Autodesk Inventor part; units mm, degrees
ref_plane "YZ Plane" through (0, 0, 0) normal (1, 0, 0) x (0, 1, 0)
ref_plane "XZ Plane" through (0, 0, 0) normal (0, 1, 0) x (-1, 0, 0)
ref_plane "XY Plane" through (0, 0, 0) normal (0, 0, 1) x (1, 0, 0)
sketch "Sketch1" plane through (0, 0, 0) normal (0, 1, 0) x (-1, 0, 0)
  line L0 (54.6051, -28.5788) -> (-2.5526, -61.5788)
  line L1 (-52.0526, -33) -> (-52.0526, 33)
  line L2 (-2.5526, 61.5788) -> (54.6051, 28.5788)
  circle A0 centre (38.1051, 0) radius 33 construction
  circle A1 centre (-19.0526, 33) radius 33 construction
  circle A2 centre (-19.0526, -33) radius 33 construction
  arc A3 (54.6051, -28.5788) -> (54.6051, 28.5788) centre (38.1051, 0) ccw
  arc A4 (-52.0526, -33) -> (-2.5526, -61.5788) centre (-19.0526, -33) ccw
  arc A5 (-2.5526, 61.5788) -> (-52.0526, 33) centre (-19.0526, 33) ccw
  circle A6 centre (0, 0) radius 3.175
  line L3 (-52.0526, -4.875) -> (-48.6526, -4.875)
  line L4 (-48.6526, -4.875) -> (-40.9371, -1.3266)
  line L5 (-40.9371, 1.3266) -> (-48.6526, 4.875)
  line L6 (-48.6526, 4.875) -> (-52.0526, 4.875)
  arc A7 (-40.9371, -1.3266) -> (-40.9371, 1.3266) centre (-38.0526, 0) ccw
  line L7 (-40.9371, -1.3266) -> (-38.0526, 0) construction
  line L8 (-38.0526, 0) -> (-40.9371, 1.3266) construction
  arc A8 (21.6175, -34.7893) -> (19.3197, -36.1159) centre (19.0263, -32.9545) ccw
  arc A9 (19.3197, 36.1159) -> (21.6175, 34.7893) centre (19.0263, 32.9545) ccw
  circle A10 centre (19.0263, 32.9545) radius 3.175
  circle A11 centre (19.0263, -32.9545) radius 3.175
  point P0 (-52.0526, 0)
  point P1 (-52.0526, 0)
  point P2 (21.6175, -34.7893)
  point P3 (21.6175, 34.7893)
  dimension "d1" = 66
  dimension "d14" = 6.35
  dimension "d15" = 9.75
  dimension "d16" = 3.4
  dimension "d18" = 10.6
  dimension "d20" = 6.35
  dimension "d23" = 360
extrude "Extrusion1" add sketch "Sketch1" along normal blind 9.525 contours L0 A4 L1 L3 L4 A7 L5 L6 A5 L2 A3
sketch "Sketch2" plane through (0, 9.525, 0) normal (0, 1, 0) x (1, 0, 0)
  circle A0 centre (19.0526, -33) radius 28.575
  circle A1 centre (-38.1051, 0) radius 28.575
  circle A2 centre (19.0526, 33) radius 28.575
  circle A3 centre (19.0526, 33) radius 33
  circle A4 centre (-38.1051, 0) radius 33
  circle A5 centre (19.0526, -33) radius 33
  line L0 (-54.6051, -28.5788) -> (2.5526, -61.5788)
  line L1 (2.5526, 61.5788) -> (-54.6051, 28.5788)
  line L2 (52.0526, -33) -> (52.0526, 33)
  point P0 (0, 0)
  point P1 (-99.3426, -2.7496)
  point P2 (47.2901, -87.408)
  point P3 (47.2901, 87.408)
  point P4 (-99.3426, 2.7496)
  point P5 (52.0526, -84.6584)
  point P6 (52.0526, 84.6584)
  dimension "d5" = 57.15
extrude "Extrusion2" cut sketch "Sketch2" against normal blind 5 contours A0 | A1 | A2
fillet "Fillet2" radius 6.35 4 edges at (52.0526, 4.7625, -4.875) (52.0526, 4.7625, 4.875) (40.9371, 4.7625, -1.3266) (40.9371, 4.7625, 1.3266)
properties part number "BOTTOM_PLATE_WEIGHTS_TREBUCHET" material "Wood (Birch)"
For this review, take the finished solid that the model builds, in its own axes (mm). A direction names the side the tool comes from. Coordinates: 2 decimals unless noted, no trailing zeros. Write each loop counter-clockwise with the first axis right and the second up, starting at its lowest first coordinate (ties: lowest second). Pieces come first, ordered by that corner, then holes. Notation, with made-up numbers: (-22, 23) - (-18, 23) arc R28 ccw to (-18, 52) - close; hole circle Ø9 at (33.5, 88). An arc over 180 degrees is marked (long way). Put each result on its own line as item: value.
1. Add section B-B, the plane x = 0. Give the boundary of the cut face in (y, z) (3 decimals), then the cut area to 3 significant figures.
Values found:
outline: (0, -60.105) - (9.525, -60.105) - (9.525, -54.296) - (4.525, -54.296) - (4.525, -11.704) - (9.525, -11.704) - (9.525, -3.175) - (0, -3.175) - close; (0, 3.175) - (9.525, 3.175) - (9.525, 11.704) - (4.525, 11.704) - (4.525, 54.296) - (9.525, 54.296) - (9.525, 60.105) - (0, 60.105) - close
area: 659 mm²
2. Mouldability with a two-part tool opening along X and no side actions: class faces 4 (the cylindrical face through (-66.652, 7.06, -1.256)), 5 (the flat face through (-5, 9.525, 0)), 6 (the flat face through (19, 4.525, 33)), 7 (the flat face through (46.607, 4.696, -3.934)) as released by +X, released by -X, zero draft, split by the parting line, or undercut.
Values found:
face 4: undercut
face 5: zero draft
face 6: undercut
face 7: released by +X
3. Wall thickness on probe 1 along X at (y, z) = (8, 33); probe 2 along Z at (x, y) = (16.5, 8); probe 3 along Z at (x, y) = (10.5, 4.75): over which ranges is each line inside the solid? List them lowest first.
Values found:
probe 1: -46.95 to -22.2, -15.85 to -9.52, 47.63 to 52.05
probe 2: -65.9 to -61.46, -4.54 to 4.54, 61.46 to 65.9
probe 3: -64.87 to -60.27, -5.73 to 5.73, 60.27 to 64.87
4. Add section D-D, the plane z = -17.5. Give the boundary of the cut face in (x, y) (1 decimal), then the cut area to 3 significant figures.
Values found:
outline: (-66.1, 0) - (52.1, 0) - (52.1, 9.5) - (43.1, 9.5) - (43.1, 4.5) - (-5, 4.5) - (-5, 9.5) - (-15.5, 9.5) - (-15.5, 4.5) - (-60.7, 4.5) - (-60.7, 9.5) - (-66.1, 9.5) - close
area: 659 mm²
5. For pin 1 (7.5 mm diameter, centred on x = -19.03, z = 32.95, fed in from -Y); pin 2 (4 mm diameter, centred on y = 7, z = -11, fed in from -X); pin 3 (5 mm diameter, centred on y = 2, z = 6.5, fed in from -X); pin 4 (4 mm diameter, centred on x = -36, y = 3, fed in from -Z), all flat-tipped, find the tip position at first contact; note any pin that passes through.
Values found:
pin 1: y = 0
pin 2: x = -69.85
pin 3: x = -70.86
pin 4: z = -40.48
6. Machinability: for faces 1 (the flat face through (-39, 4.525, 0)), 2 (the cylindrical face through (41.954, 4.696, -2.386)), 3 (the flat face through (46.55, 4.7, 3.91)), which of the approach directions +Z, -Z, +X, -X, +Y, -Y give a long, thin tool a straight path to every point of the face, cutting with its end or side? Answer none if there is none.
Values found:
face 1: +Y
face 2: +Y, -Y
face 3: +X, +Y, -Y
7. Add section C-C, the plane y = 8. Count the separate pieces of the cut face and the enclosed holes in it, then the cut area to 3 significant figures.
Values found:
separate pieces: 1
enclosed holes: 6
area: 3,920 mm²
8. Add section A-A, the plane z = 0. Give the boundary of the cut face in (x, y) (3 decimals).
Values found:
outline: (-71.105, 0) - (-3.175, 0) - (-3.175, 9.525) - (-9.53, 9.525) - (-9.53, 4.525) - (-66.68, 4.525) - (-66.68, 9.525) - (-71.105, 9.525) - close; (3.175, 0) - (34.878, 0) - (34.878, 9.525) - (3.175, 9.525) - close
